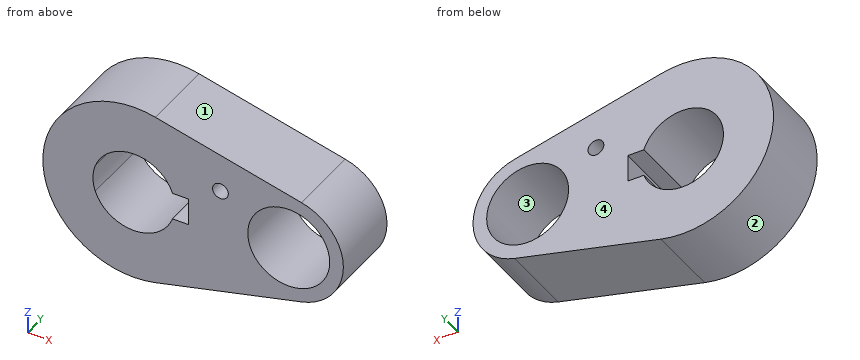
```python
from build123d import *

# Parameters (mm, degrees)
F0_R     = 14.2875
F1_DEPTH = 25.4
F3_D     = 5.5


with BuildPart() as f1:
    # F0 (on Front) → F1 (new body)
    with BuildSketch(Plane.XZ):
        with BuildLine():
            ThreePointArc((7.4705882353, -30.8585938017), (24.9524916238, -19.6325154212), (31.75, 0))
            ThreePointArc((31.75, 0), (24.9524916238, 19.6325154212), (7.4705882353, 30.8585938017))
            ThreePointArc((7.4705882353, 30.8585938017), (-31.75, 0), (7.4705882353, -30.8585938017))
        make_face()
        with BuildLine():
            ThreePointArc((-13.4703841816, 4.7625), (0, 14.2875), (13.4703841816, 4.7625))
            Line((13.4703841816, 4.7625), (19.05, 4.7625))
            Line((19.05, 4.7625), (19.05, -4.7625))
            Line((19.05, -4.7625), (13.4703841816, -4.7625))
            ThreePointArc((13.4703841816, -4.7625), (0, -14.2875), (-13.4703841816, -4.7625))
            Line((-13.4703841816, -4.7625), (-19.05, -4.7625))
            Line((-19.05, -4.7625), (-19.05, 4.7625))
            Line((-19.05, 4.7625), (-13.4703841816, 4.7625))
        make_face(mode=Mode.SUBTRACT)
        with BuildLine():
            ThreePointArc((-13.4703841816, -4.7625), (-14.2875, 0), (-13.4703841816, 4.7625))
            Line((-13.4703841816, 4.7625), (-19.05, 4.7625))
            Line((-19.05, 4.7625), (-19.05, -4.7625))
            Line((-19.05, -4.7625), (-13.4703841816, -4.7625))
        make_face()
        with BuildLine():
            ThreePointArc((7.4705882353, 30.8585938017), (24.9524916238, 19.6325154212), (31.75, 0))
            ThreePointArc((31.75, 0), (24.9524916238, -19.6325154212), (7.4705882353, -30.8585938017))
            Line((7.4705882353, -30.8585938017), (58.4573529412, -18.515156281))
            ThreePointArc((58.4573529412, -18.515156281), (34.925, 0), (58.4573529412, 18.515156281))
            Line((58.4573529412, 18.515156281), (7.4705882353, 30.8585938017))
        make_face()
        with BuildLine():
            ThreePointArc((73.025, 0), (68.9464949743, 11.7795092527), (58.4573529412, 18.515156281))
            ThreePointArc((58.4573529412, 18.515156281), (34.925, 0), (58.4573529412, -18.515156281))
            ThreePointArc((58.4573529412, -18.515156281), (68.9464949743, -11.7795092527), (73.025, 0))
        make_face()
        with Locations((53.975, 0)):
            Circle(F0_R, mode=Mode.SUBTRACT)
    extrude(amount=F1_DEPTH)

    # F3 (through all)
    with Locations(Plane.XZ.offset(25.4)):
        with Locations((30.1617980003, 11.9795044884)):
            Hole(F3_D / 2)


solid = f1.part
```
For this review, take the finished solid that the model builds, in its own axes (mm). Face numbers are marked on the shaded views. Round coordinates to 2 decimals unless told otherwise and drop trailing zeros. Write each loop counter-clockwise with the first axis right and the second up, starting at its lowest first coordinate (ties: lowest second). Pieces come first, ordered by that corner, then holes.
1) Take a section at D-D on x = 11.5. Give the boundary of the cut face in (y, z), then the cut area to 3 significant figures.
Answer below:
outline: (-25.4, -29.88) - (0, -29.88) - (0, -8.48) - (-25.4, -8.48) - close; (-25.4, 8.48) - (0, 8.48) - (0, 29.88) - (-25.4, 29.88) - close
area: 1,090 mm2
2) Mouldability with a two-part tool opening along X and no side actions: class the marked faces 1, 2, 3 and 4 as +X half, -X half, draft (parallel to the pull), parting line (faces both ways), or undercut.
Answer below:
face 1: +X half
face 2: parting line
face 3: undercut
face 4: draft
3) Take a section at A-A on z = 0. State how many separate pieces and enclosed holes the cut face has, then the cut area to 3 significant figures.
Answer below:
separate pieces: 3
enclosed holes: 0
area: 1,090 mm2
4) For line 1 along X through (y, z) = (-24, 3.5); line 2 along X through (y, z) = (-14, -1); line 3 along Z through (x, y) = (42.5, -7), list the stretches that pass through material, from the lowest coordinate up.
Answer below:
line 1: x = -31.56 to -13.85, 19.05 to 40.12, 67.83 to 72.7
line 2: x = -31.73 to -14.25, 19.05 to 39.72, 68.23 to 73
line 3: z = -22.38 to -8.51, 8.51 to 22.38
5) Insertion check: pin 1 Ø1.5 at (x, y) = (52.5, -12) entering from +Z; pin 2 Ø3 at (y, z) = (-16.5, 18) entering from -X; pin 3 Ø4.5 at (x, y) = (15.5, -14.5) entering from -Z. Each pin has a flat end and moves straight along its axis. Give the tip position at first contact, or say it passes through.
Answer below:
pin 1: stops at z = 20.14
pin 2: stops at x = -27.13
pin 3: stops at z = -29.46
6) Take a section at B-B on x = 0. Give the boundary of the cut face in (y, z), then the cut area to 3 significant figures.
Answer below:
outline: (-25.4, -31.75) - (0, -31.75) - (0, -14.29) - (-25.4, -14.29) - close; (-25.4, 14.29) - (0, 14.29) - (0, 31.75) - (-25.4, 31.75) - close
area: 887 mm2
